CAD build for the part. Positions are in the model's coordinates, mm. Face numbers are marked on the shaded views. A direction names the side the tool comes from. Give positions to 0.01 mm unless a question says otherwise; leave off trailing zeros. Loops run counter-clockwise (first coordinate to the right, second up) from the corner with the lowest first, then second, coordinate; pieces in that order, holes last.
Item 1: Drop flat-ended pins along their axis: P1, Ø12, axis at y = 23, z = 49.5, coming from the +X side; P2, Ø19.5, axis at y = -19.5, z = 16, coming from the +X side; P3, Ø1.5, axis at x = 79, z = 84, coming from the +Y side. Give the stop position or say it passes through.
Item 2: Probe probe 1 along Z at (x, y) = (31, -38.5); probe 2 along Z at (x, y) = (69.5, 2); probe 3 along Y at (x, z) = (-21, 19). List the from-to ranges inside material, lowest first.
Item 3: Which spindle directions (+Z, -Z, +X, -X, +Y, -Y) get a long thin tool onto all of the face, cutting with end or side? Do the marked faces 1, 2, 3 and 4. Say none if no direction does.
Item 4: Saw through at B-B on y = 18. Give the cut face in (x, z).
Item 5: Saw through at C-C on x = 95. Give the cut face in (y, z) (3 decimals), plus the area to 3 significant figures.
Item 6: Saw through at A-A on y = 31.5. Give the cut face in (x, z), plus the area to 3 significant figures.
Item 7: Mould opens along X. For the marked faces 5, 6, 7 and 8 say: released by +X, released by -X, zero draft, split by the parting line, or undercut.
Item 8: Saw through at D-D on x = 72. Give the cut face in (y, z), plus the area to 3 significant figures.
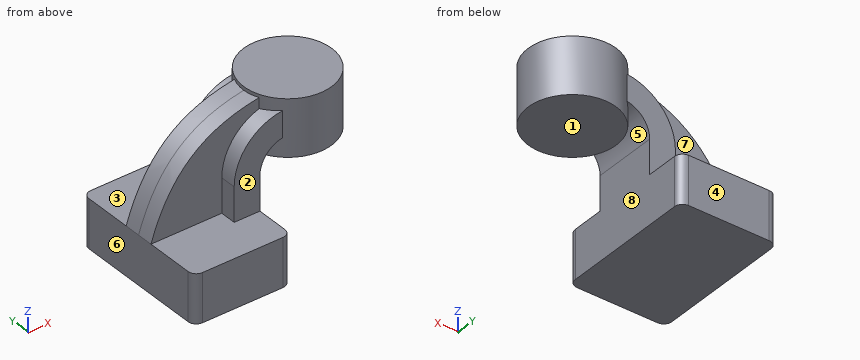
from build123d import *

# Parameters (mm, degrees)
F1_DEPTH = 57.15
F2_DEPTH = 25.4
F3_DEPTH = 12.7
F0_W     = 34.6883076322
F0_H     = 8.9280228981
F0_H_2   = 20.32
F0_H_3   = 15.2019771019
F5_R     = 6.35


with BuildPart() as f1:
    # F0 (on Front) → F1 (new body, symmetric)
    with BuildSketch(Plane.XZ):
        Polygon((-34.9306485406, 17.8198447397), (-34.9306485406, -20.2801552603), (41.2693514594, -20.2801552603), (41.2693514594, 17.8198447397), (20.9493514594, 17.8198447397), align=None)
    extrude(amount=F1_DEPTH, both=True)

    # F0 (on Front) → F2 (join, symmetric)
    with BuildSketch(Plane.XZ):
        with BuildLine():
            Line((20.9493514594, 17.8198447397), (41.2693514594, 17.8198447397))
            Line((41.2693514594, 17.8198447397), (41.2693514594, 44.7438447397))
            ThreePointArc((41.2693514594, 44.7438447397), (47.5929160536, 60.0102801456), (62.8593514594, 66.3338447397))
            Line((62.8593514594, 66.3338447397), (82.7810438272, 66.3338447397))
            Line((82.7810438272, 66.3338447397), (82.7810438272, 86.6538447397))
            Line((82.7810438272, 86.6538447397), (62.8593514594, 86.6538447397))
            ThreePointArc((62.8593514594, 86.6538447397), (33.2245062599, 74.3786899393), (20.9493514594, 44.7438447397))
            Line((20.9493514594, 44.7438447397), (20.9493514594, 17.8198447397))
        make_face()
    extrude(amount=F2_DEPTH, both=True)

    # F0 (on Front) → F3 (join, symmetric)
    with BuildSketch(Plane.XZ):
        with BuildLine():
            add(Edge.make_bspline(
                [(82.7810438272, 95.5818676378), (25.6006252021, 94.6536809206), (-14.9303628132, 80.6806907058), (-34.9306485406, 17.8198447397)],
                knots=[0, 0, 0, 0, 141.0779030369, 141.0779030369, 141.0779030369, 141.0779030369], degree=3))
            Line((-34.9306485406, 17.8198447397), (20.9493514594, 17.8198447397))
            Line((20.9493514594, 17.8198447397), (20.9493514594, 44.7438447397))
            ThreePointArc((20.9493514594, 44.7438447397), (33.2245062599, 74.3786899393), (62.8593514594, 86.6538447397))
            Line((62.8593514594, 86.6538447397), (82.7810438272, 86.6538447397))
            Line((82.7810438272, 86.6538447397), (82.7810438272, 95.5818676378))
        make_face()
    extrude(amount=F3_DEPTH, both=True)

    # F0 (on Front) → F4 (revolve)
    with BuildSketch(Plane.XZ):
        with Locations((100.1251976433, 91.1178561888)):
            Rectangle(F0_W, F0_H)
        with Locations((100.1251976433, 76.4938447397)):
            Rectangle(F0_W, F0_H_2)
        with Locations((100.1251976433, 58.7328561888)):
            Rectangle(F0_W, F0_H_3)
    revolve(axis=Axis((82.7810438272, 0, 73.3568676378), (0, 0, -1)))

    # F5
    f5_edges = [f1.edges().sort_by_distance(p)[0] for p in [
        (41.269351, 57.15, -1.230155),
        (-34.930649, 57.15, -1.230155),
        (41.269351, -57.15, -1.230155),
        (-34.930649, -57.15, -1.230155),
    ]]
    fillet(f5_edges, radius=F5_R)


solid = f1.part
Results below:
1. P1: stops at x = 112.89
1. P2: stops at x = 41.27
1. P3: stops at y = 34.56
2. probe 1: z = -20.28 to 17.82
2. probe 2: z = 51.13 to 95.58
2. probe 3: y = -12.7 to 12.7
3. face 1: -Z, +X, +Y, -Y
3. face 2: +Z, -X, -Y
3. face 3: +Z, -X, +Y
3. face 4: +Z, -Z, +X, -X, +Y
4. outline: (-34.93, -20.28) - (41.27, -20.28) - (41.27, 44.74) arc R21.59 cw to (53.13, 64.02) - (53.13, 51.13) - (112.43, 51.13) - (112.43, 95.58) - (53.13, 95.58) - (53.13, 85.51) arc R41.91 ccw to (20.95, 44.74) - (20.95, 17.82) - (-34.93, 17.82) - close
5. outline: (-32.465, 51.132) - (32.465, 51.132) - (32.465, 95.582) - (-32.465, 95.582) - close
5. area: 2,890 mm2
6. outline: (-34.93, -20.28) - (41.27, -20.28) - (41.27, 17.82) - (-34.93, 17.82) - close; (68.25, 51.13) - (97.31, 51.13) - (97.31, 95.58) - (68.25, 95.58) - close
6. area: 4,190 mm2
7. face 5: undercut
7. face 6: released by -X
7. face 7: zero draft
7. face 8: released by +X
8. outline: (-32.97, 51.13) - (32.97, 51.13) - (32.97, 95.58) - (-32.97, 95.58) - close
8. area: 2,930 mm2
